Autodesk Inventor part; units mm, degrees
ref_plane "YZ Plane" through (0, 0, 0) normal (1, 0, 0) x (0, 1, 0)
ref_plane "XZ Plane" through (0, 0, 0) normal (0, 1, 0) x (-1, 0, 0)
ref_plane "XY Plane" through (0, 0, 0) normal (0, 0, 1) x (1, 0, 0)
sketch "Sketch1" plane through (0, 0, 0) normal (0, 1, 0) x (-1, 0, 0)
  line L0 (600, 0) -> (600, -30)
  arc A0 (545.3858, -119.1074) -> (600, -30) centre (500, -30) ccw
  arc A1 (0, -250) -> (545.3858, -119.1074) centre (0, 951.6667) ccw
  line L1 (0, 191.6842) -> (0, -191.6842)
  arc A2 (0, -244) -> (542.6626, -113.761) centre (0, 951.6667) ccw
  arc A3 (542.6626, -113.761) -> (594, -30) centre (500, -30) ccw
  line L2 (594, -30) -> (594, 0)
  line L3 (594, 0) -> (600, 0)
  line L4 (0, -244) -> (0, -250)
  point P0 (0, 0)
  point P1 (0, 0)
  point P2 (0, -247)
  point P3 (0, -163.7009)
  point P4 (0, -169.7009)
  dimension "d0" = 100
  dimension "d1" = 30
  dimension "d3" = 1201.6667
  dimension "d6" = 6
  dimension "d11" = 1188
  dimension "d12" = 250
revolve "Revolution1" add sketch "Sketch1" angle 360 about axis through (0, 0, 191.6842) along (0, 0, -1)
sketch "Sketch2" plane through (0, 0, 0) normal (0, 0, 1) x (1, 0, 0)
  circle A0 centre (0, 0) radius 16.75
  dimension "d8" = 33.5
extrude "Extrusion1" cut sketch "Sketch2" against normal through all
equation "\"d11\" = MAIN_filter_diam"
equation "\"MAIN_filter_diam\" = 1188"
equation "\"Disherd_head_hight\" = d12"
properties part number "PNS 1604 dished head D1000_1200"
For this review, take the finished solid that the model builds, in its own axes (mm). Give positions to 0.01 mm unless a question says otherwise; leave off trailing zeros. Loops run counter-clockwise (first coordinate to the right, second up) from the corner with the lowest first, then second, coordinate; pieces in that order, holes last. Notation, with made-up numbers: M 61,-28 L 120,-28 A21 cw 120,-20 Z; hole C 76,86.5 d6. An arc over 180 degrees is marked long. One line per item, written item: value. Start each with the question number.
Q1. For L1, parallel to Y at x = 0, z = -9.75; L2, parallel to X at y = 351, z = -54.5; L3, parallel to X at y = -385.5, z = -62, list the stretches that pass through material, from the lowest coordinate up.
Q2. Clearance check with flat-ended pins moving along their axes: pin 1 Ø12 at (x, z) = (257, -93.5) entering from +Y; pin 2 Ø1 at (x, z) = (-187.5, -36.5) entering from +Y; pin 3 Ø6 at (y, z) = (-28, -113) entering from +X. State where each tip first meets the part, or that it passes through.
Q3. Draft analysis for pull direction X (two halves, no side actions). For faces 1 (the face through (78.108, 594.894, -15.21)), 2 (the face through (581, 136, 0)), 3 (the face through (77.327, -588.945, -14.79)), state which applies: released by +X, released by -X, zero draft, split by the parting line, or undercut.
Q4. Add section A-A (z = -84.5). Give the boundary of the cut face in (x, y), and give its area (3 significant figures).
Reply:
1. L1: -600 to -594, 594 to 600
1. L2: -482.86 to -475.17, 475.17 to 482.86
1. L3: -452.89 to -444.51, 444.51 to 452.89
2. pin 1: y = 522.81
2. pin 2: y = 569.9
2. pin 3: x = 559.3
3. face 1: split by the parting line
3. face 2: zero draft
3. face 3: undercut
4. outline: C 0,0 d1167.69; hole C 0,0 d1153.18
4. area: 26,500 mm²
